Work out the finished part from the listing and answer in its coordinate system (mm). Round coordinates to 2 decimals unless told otherwise and drop trailing zeros. Order: outer loops, then holes, each group sorted by start corner. A loop starts at its lowest first (then second) coordinate and runs counter-clockwise, first axis right, second up. Notation, with made-up numbers: (49.25, 79) - (70.25, 79) arc R34 ccw to (70.25, 112) - close; hole circle Ø2 at (-8.75, 88.25). An arc over 180 degrees is marked (long way). Answer in a Markdown table with one row per item.
Solid Edge part; units mm, degrees
sketch "Sketch1" plane through (0, 0, 0) normal (0, -1, 0) x (1, 0, 0)
  arc A0 (-1.9633, 10.292) -> (0.6579, 10.4569) centre (-1.4017, 22.2789) ccw
  arc A1 (0.6579, 10.4569) -> (3.2378, 9.9648) centre (4.1829, 21.9275) ccw
  arc A2 (3.2378, 9.9648) -> (5.6142, 8.8465) centre (9.5046, 20.1984) ccw
  arc A3 (5.6142, 8.8465) -> (7.6378, 7.1724) centre (14.2292, 17.2001) ccw
  arc A4 (7.6378, 7.1724) -> (9.1816, 5.0476) centre (18.0596, 13.1211) ccw
  arc A5 (9.1816, 5.0476) -> (10.1484, 2.6057) centre (20.7553, 8.2176) ccw
  arc A6 (10.1484, 2.6057) -> (10.1484, -0.4889) centre (17.4001, 1.0584) ccw
  arc A7 (10.1484, -0.4889) -> (10.1484, -3.095) centre (13.9226, -1.792) ccw
  arc A8 (10.1484, -3.095) -> (9.1816, -5.0476) centre (12.6667, -5.5576) ccw
  arc A9 (9.1816, -5.0476) -> (7.6378, -7.1724) centre (18.0596, -13.1211) ccw
  arc A10 (7.6378, -7.1724) -> (5.6142, -8.8465) centre (14.2292, -17.2001) ccw
  arc A11 (5.6142, -8.8465) -> (3.2378, -9.9648) centre (9.5046, -20.1984) ccw
  arc A12 (3.2378, -9.9648) -> (0.6579, -10.4569) centre (4.1829, -21.9275) ccw
  arc A13 (0.6579, -10.4569) -> (-1.9633, -10.292) centre (-1.4017, -22.2789) ccw
  arc A14 (-1.9633, -10.292) -> (-4.4611, -9.4804) centre (-6.8982, -21.2303) ccw
  arc A15 (-4.4611, -9.4804) -> (-6.6787, -8.0731) centre (-11.9612, -18.8479) ccw
  arc A16 (-6.6787, -8.0731) -> (-8.4766, -6.1586) centre (-16.2727, -15.2811) ccw
  arc A17 (-8.4766, -6.1586) -> (-9.7418, -3.8571) centre (-19.5617, -10.7541) ccw
  arc A18 (-9.7418, -3.8571) -> (-10.395, -1.3132) centre (-21.6216, -5.5515) ccw
  arc A19 (-10.395, -1.3132) -> (-10.395, 1.3132) centre (-22.3229, 0) ccw
  arc A20 (-10.395, 1.3132) -> (-9.7418, 3.8571) centre (-21.6216, 5.5515) ccw
  arc A21 (-9.7418, 3.8571) -> (-8.4766, 6.1586) centre (-19.5617, 10.7541) ccw
  arc A22 (-8.4766, 6.1586) -> (-6.6787, 8.0731) centre (-16.2727, 15.2811) ccw
  arc A23 (-6.6787, 8.0731) -> (-4.4611, 9.4804) centre (-11.9612, 18.8479) ccw
  arc A24 (-4.4611, 9.4804) -> (-1.9633, 10.292) centre (-6.8982, 21.2303) ccw
  circle A25 centre (0, 0) radius 8.8442
extrude "Protrusion1" add sketch "Sketch1" against normal blind 600
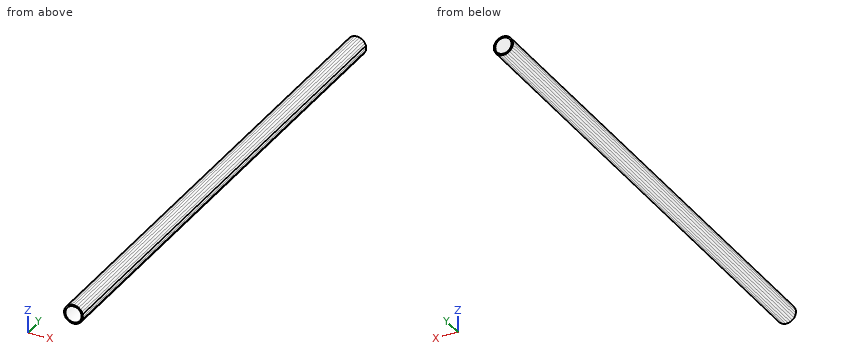
1) Each of these flat-tipped pins is pushed along its axis until it touches: pin 1 (1.5 mm diameter, centred on y = 487, z = 4, fed in from +X); pin 2 (2 mm diameter, centred on x = 4.5, z = -8, fed in from -Y); pin 3 (1.5 mm diameter, centred on x = -5.5, y = 400, fed in from -Z). Where does it stop, or does it pass through?
Filled in:
| item | result |
|---|---|
| pin 1 | stops at x = 9.83 |
| pin 2 | stops at y = 0 |
| pin 3 | stops at z = -9.26 |
2) Find section A-A, the plane y = 364. Give the vertices of the cut face in (x, z) (1 decimal).
Filled in:
| item | result |
|---|---|
| outline | (-10.4, -1.3) arc R12 cw to (-9.7, -3.9) arc R12 cw to (-8.5, -6.2) arc R12 cw to (-6.7, -8.1) arc R12 cw to (-4.5, -9.5) arc R12 cw to (-2, -10.3) arc R12 cw to (0.7, -10.5) arc R12 cw to (3.2, -10) arc R12 cw to (5.6, -8.8) arc R12 cw to (7.6, -7.2) arc R12 cw to (9.2, -5) arc R3.5 cw to (10.1, -3.1) arc R4 cw to (10.1, -0.5) arc R7.4 cw to (10.1, 2.6) arc R12 cw to (9.2, 5) arc R12 cw to (7.6, 7.2) arc R12 cw to (5.6, 8.8) arc R12 cw to (3.2, 10) arc R12 cw to (0.7, 10.5) arc R12 cw to (-2, 10.3) arc R12 cw to (-4.5, 9.5) arc R12 cw to (-6.7, 8.1) arc R12 cw to (-8.5, 6.2) arc R12 cw to (-9.7, 3.9) arc R12 cw to (-10.4, 1.3) arc R12 cw to start; hole circle Ø17.7 at (0, 0) |
3) Find the intervals of material crossed by probe 1 along Z at (x, y) = (0, 322); probe 2 along X at (y, z) = (148, 1.5); probe 3 along Z at (x, y) = (4.75, 493.5), in increasing order. Write a range as from..to.
Filled in:
| item | result |
|---|---|
| probe 1 | z = -10.36..-8.84, 8.84..10.36 |
| probe 2 | x = -10.33..-8.72, 8.72..10 |
| probe 3 | z = -9.18..-7.46, 7.46..9.18 |
